Check sheet for the modelled part. Datum: model origin and axes. Units: mm. Coordinates: 2 decimals unless noted, no trailing zeros. Loops run counter-clockwise (first coordinate to the right, second up) from the corner with the lowest first, then second, coordinate; pieces in that order, holes last. Notation, with made-up numbers: M 44.25,77.5 L 86.25,77.5 A15 cw 86.25,99.5 Z; hole C 20.25,67 d3. An arc over 180 degrees is marked long. Write each question's results on one line, items separated by ' | '. Start each with the question number.
from build123d import *

# Parameters (mm, degrees)
SKETCH1_W                 = 101.6
SKETCH1_H                 = 38.1
SKETCH1_R                 = 9.017
BOSS_EXTRUDE1_DEPTH       = 4.7625
F_4_CLEARANCE_HOLE1_D     = 3.2639
F_4_CLEARANCE_HOLE1_DEPTH = 25.4
F_4_CLEARANCE_HOLE1_TIP   = 0.980574487
FILLET1_R                 = 12.7


with BuildPart() as part:
    # Sketch1 → Boss-Extrude1 (new body)
    with BuildSketch(Plane(origin=(0, 0, 0), x_dir=(1, 0, 0), z_dir=(0, 1, 0))):
        with Locations((50.8, 19.05)):
            Rectangle(SKETCH1_W, SKETCH1_H)
        with Locations((25.4, 19.05)):
            Circle(SKETCH1_R, mode=Mode.SUBTRACT)
        with Locations((76.2, 19.05)):
            Circle(SKETCH1_R, mode=Mode.SUBTRACT)
    extrude(amount=BOSS_EXTRUDE1_DEPTH)

    # #4 Clearance Hole1
    with Locations(Plane(origin=(0, 4.7625, 0), x_dir=(-1, 0, 0), z_dir=(0, 1, 0))):
        with Locations((-25.4, -29.845), (-36.195, -19.05), (-25.4, -8.255), (-14.605, -19.05), (-65.405, -19.05), (-76.2, -29.845), (-86.995, -19.05), (-76.2, -8.255)):
            Hole(F_4_CLEARANCE_HOLE1_D / 2, depth=F_4_CLEARANCE_HOLE1_DEPTH)
            with Locations((0, 0, -(F_4_CLEARANCE_HOLE1_DEPTH + F_4_CLEARANCE_HOLE1_TIP / 2))):  # 118° drill point
                Cone(0, F_4_CLEARANCE_HOLE1_D / 2, F_4_CLEARANCE_HOLE1_TIP, mode=Mode.SUBTRACT)

    # Fillet1
    fillet1_edges = [part.edges().sort_by_distance(p)[0] for p in [
        (0, 2.38125, -38.1),
        (101.6, 2.38125, -38.1),
        (101.6, 2.38125, 0),
        (0, 2.38125, 0),
    ]]
    fillet(fillet1_edges, radius=FILLET1_R)


solid = part.part
Item 1: Section check A-A (x = 76.2). Record the cut outline in (y, z), plus the area to 3 significant figures.
Item 2: Thickness scan on line 1 (Z direction, x = 25.5, y = 3); line 2 (X direction, y = 1.5, z = -26); line 3 (X direction, y = 1.65, z = -13). Record the ranges inside material, lowest first.
Item 3: Section check C-C (x = 19). Record the cut outline in (y, z), plus the area to 3 significant figures.
Item 4: Section check D-D (y = 1.15). State how many separate pieces and enclosed holes the cut face has, plus the area to 3 significant figures.
Item 5: Section check B-B (z = -19.05). Record the cut outline in (x, y).
Item 6: Release check for a two-part mould opening along X. For faces 1 (the face through (50, 0, -19)), 2 (the face through (66.9, 2.3, -19.7)), 3 (the face through (101.6, 2, -19)) record: +X half, -X half, draft (parallel to the pull), parting line (faces both ways), or undercut.
Item 7: Depth check by flat-ended pin: P1, Ø1.5, axis at y = 1, z = -31, coming from the +X side; P2, Ø1, axis at x = 65, z = -19.5, coming from the +Y side. Enter the tip coordinate at first touch or a pass-through.
Computed values:
1) outline: M 0,-38.1 L 4.76,-38.1 L 4.76,-31.48 L 0,-31.48 Z; M 0,-28.21 L 4.76,-28.21 L 4.76,-28.07 L 0,-28.07 Z; M 0,-10.03 L 4.76,-10.03 L 4.76,-9.89 L 0,-9.89 Z; M 0,-6.62 L 4.76,-6.62 L 4.76,0 L 0,0 Z | area: 64.5 mm²
2) line 1: z = -38.1 to -31.47, -28.22 to -28.07, -10.03 to -9.88, -6.63 to 0 | line 2: x = 0.01 to 19.66, 31.14 to 70.46, 81.94 to 101.59 | line 3: x = 0 to 18.71, 32.09 to 69.51, 82.89 to 101.6
3) outline: M 0,-38.1 L 4.76,-38.1 L 4.76,-25.4 L 0,-25.4 Z; M 0,-12.7 L 4.76,-12.7 L 4.76,0 L 0,0 Z | area: 121 mm²
4) separate pieces: 1 | enclosed holes: 10 | area: 3,150 mm²
5) outline: M 0,0 L 12.97,0 L 12.97,4.76 L 0,4.76 Z; M 16.24,0 L 16.38,0 L 16.38,4.76 L 16.24,4.76 Z; M 34.42,0 L 34.56,0 L 34.56,4.76 L 34.42,4.76 Z; M 37.83,0 L 63.77,0 L 63.77,4.76 L 37.83,4.76 Z; M 67.04,0 L 67.18,0 L 67.18,4.76 L 67.04,4.76 Z; M 85.22,0 L 85.36,0 L 85.36,4.76 L 85.22,4.76 Z; M 88.63,0 L 101.6,0 L 101.6,4.76 L 88.63,4.76 Z
6) face 1: draft | face 2: undercut | face 3: +X half
7) P1: stops at x = 100.64 | P2: passes through
